```python
from build123d import *

# Parameters (mm, degrees)
SKETCH1_R           = 1.4
BOSS_EXTRUDE1_DEPTH = 2
BOSS_EXTRUDE2_DEPTH = 6


with BuildPart() as part:
    # Sketch1 → Boss-Extrude1 (new body)
    with BuildSketch(Plane.XY):
        with BuildLine():
            Line((78.466333699, 24.25), (60.234282891, 55.828838325))
            ThreePointArc((60.234282891, 55.828838325), (45.078838325, 64.578838325), (29.923393759, 55.828838325))
            Line((29.923393759, 55.828838325), (11.691342951, 24.25))
            ThreePointArc((11.691342951, 24.25), (11.594517635, 6.919891409), (26.455726065, -1.995630053))
            ThreePointArc((26.455726065, -1.995630053), (26.732773023, -2.115865565), (26.846787517, -2.395530168))
            Line((26.846787517, -2.395530168), (26.846787517, -2.834314575))
            ThreePointArc((26.846787517, -2.834314575), (26.81633933, -2.987387948), (26.72963023, -3.117157288))
            Line((26.72963023, -3.117157288), (26.105366161, -3.741421356))
            ThreePointArc((26.105366161, -3.741421356), (26.062011611, -3.806306026), (26.046787517, -3.882842712))
            Line((26.046787517, -3.882842712), (26.046787517, -4))
            ThreePointArc((26.046787517, -4), (26.105366161, -4.141421356), (26.246787517, -4.2))
            Line((26.246787517, -4.2), (63.910889132, -4.2))
            ThreePointArc((63.910889132, -4.2), (64.052310489, -4.141421356), (64.110889132, -4))
            Line((64.110889132, -4), (64.110889132, -3.882842712))
            ThreePointArc((64.110889132, -3.882842712), (64.095665039, -3.806306026), (64.052310489, -3.741421356))
            Line((64.052310489, -3.741421356), (63.42804642, -3.117157288))
            ThreePointArc((63.42804642, -3.117157288), (63.341337319, -2.987387948), (63.310889132, -2.834314575))
            Line((63.310889132, -2.834314575), (63.310889132, -2.395530168))
            ThreePointArc((63.310889132, -2.395530168), (63.424903627, -2.115865565), (63.701950585, -1.995630053))
            ThreePointArc((63.701950585, -1.995630053), (78.563159015, 6.919891409), (78.466333699, 24.25))
        make_face()
        with Locations((65.994459855, 38.101919162)):
            Circle(SKETCH1_R, mode=Mode.SUBTRACT)
        with Locations((45.078838325, 1.875)):
            Circle(SKETCH1_R, mode=Mode.SUBTRACT)
        with Locations((24.163216795, 38.101919162)):
            Circle(SKETCH1_R, mode=Mode.SUBTRACT)
        with BuildLine():
            Line((26.846787517, 10.5), (63.310889132, 10.5))
            ThreePointArc((63.310889132, 10.5), (67.641016151, 13), (67.641016151, 18))
            Line((67.641016151, 18), (49.408965344, 49.578838325))
            ThreePointArc((49.408965344, 49.578838325), (45.078838325, 52.078838325), (40.748711306, 49.578838325))
            Line((40.748711306, 49.578838325), (22.516660498, 18))
            ThreePointArc((22.516660498, 18), (22.516660498, 13), (26.846787517, 10.5))
        make_face(mode=Mode.SUBTRACT)
    extrude(amount=BOSS_EXTRUDE1_DEPTH)

    # Sketch2 → Boss-Extrude2 (add)
    with BuildSketch(Plane(origin=(0, 0, 0), x_dir=(-1, 0, 0), z_dir=(0, 0, -1))):
        with BuildLine():
            ThreePointArc((-27.949498848, 42.516002182), (-45.078838325, 62.398838325), (-62.208177802, 42.516002182))
            ThreePointArc((-62.208177802, 42.516002182), (-63.337010114, 36.567639839), (-67.924026858, 32.615861208))
            ThreePointArc((-67.924026858, 32.615861208), (-76.578398318, 7.84), (-50.794687381, 2.946974934))
            ThreePointArc((-50.794687381, 2.946974934), (-45.078838325, 4.943558647), (-39.362989268, 2.946974934))
            ThreePointArc((-39.362989268, 2.946974934), (-13.579278331, 7.84), (-22.233649792, 32.615861208))
            ThreePointArc((-22.233649792, 32.615861208), (-26.820666536, 36.567639839), (-27.949498848, 42.516002182))
        make_face()
        with BuildLine():
            ThreePointArc((-67.623619549, 31.852870089), (-62.626869283, 36.157639839), (-61.397204455, 42.637337381))
            ThreePointArc((-61.397204455, 42.637337381), (-45.078838325, 61.578838325), (-28.760472195, 42.637337381))
            ThreePointArc((-28.760472195, 42.637337381), (-27.530807367, 36.157639839), (-22.534057101, 31.852870089))
            ThreePointArc((-22.534057101, 31.852870089), (-14.289419162, 8.25), (-38.852423231, 3.588630855))
            ThreePointArc((-38.852423231, 3.588630855), (-45.078838325, 5.763558647), (-51.305253419, 3.588630855))
            ThreePointArc((-51.305253419, 3.588630855), (-75.868257487, 8.25), (-67.623619549, 31.852870089))
        make_face(mode=Mode.SUBTRACT)
    extrude(amount=BOSS_EXTRUDE2_DEPTH)


solid = part.part
```
Geometry check sheet. Reference: the model listing, model coordinates, mm. A direction names the side the tool comes from. Coordinates: 2 decimals unless noted, no trailing zeros. Order: outer loops, then holes, each group sorted by start corner. A loop starts at its lowest first (then second) coordinate and runs counter-clockwise, first axis right, second up.
Item 1: Section check A-A (y = 16.5). Enter the section's corners in (x, z).
Item 2: Depth check by flat-ended pin: pin 1 (4 mm diameter, centred on y = 17.5, z = -1, fed in from +X); pin 2 (2 mm diameter, centred on x = 48, z = 1, fed in from +Y); pin 3 (4 mm diameter, centred on x = 53.5, y = 42.5, fed in from -Z). Enter the tip coordinate at first touch or a pass-through.
Item 3: Section check B-B (x = 37). Enter the section's corners in (y, z), plus the area to 3 significant figures.
Item 4: Mould release check, pull along Y, two halves, no side actions. Record for faces 1 (the flat face through (20.935, 40.26, 0.986)), 2 (the flat face through (29, 31, 2)), 3 (the cylindrical face through (63.294, 36.643, -2.958)): released by +Y, released by -Y, zero draft, split by the parting line, or undercut.
Item 5: Tool access check on faces 4 (the flat face through (48, 2, 0)), 5 (the cylindrical face through (67.604, 12.937, 0.986)), 6 (the cylindrical face through (45.165, 4.943, -2.958)), 7 (the cylindrical face through (78.437, 6.7, 0.986)), 8 (the cylindrical face through (11.472, 7.142, 0.986)). Record the directions out of +Z, -Z, +X, -X, +Y, -Y that give a thin tool (end or side, any length) a straight path to the whole face; none if there is none.
Item 6: Section check D-D (z = 1). Count the separate pieces of the cut face and the enclosed holes in it, plus the area to 3 significant figures.
Item 7: Section check C-C (z = -3.5). Enter the section's corners in (x, y).
Item 8: Scan lines: line 1 along X through (y, z) = (16.5, -4.05); line 2 along X through (y, z) = (3, -0.5); line 3 along X through (y, z) = (31, -1.5). Record each from-to range of solid material in increasing order.
Check sheet entries:
1. outline: (9.38, 0) - (11.26, 0) - (11.26, -6) - (12.08, -6) - (12.08, 0) - (21.95, 0) - (21.95, 2) - (9.38, 2) - close; (68.21, 0) - (78.08, 0) - (78.08, -6) - (78.9, -6) - (78.9, 0) - (80.78, 0) - (80.78, 2) - (68.21, 2) - close
2. pin 1: stops at x = 80.81
2. pin 2: stops at y = 64.47
2. pin 3: stops at z = 0
3. outline: (-4.2, 0) - (1.37, 0) - (1.37, -6) - (2.31, -6) - (2.31, 0) - (10.5, 0) - (10.5, 2) - (-4.2, 2) - close; (43.09, 0) - (59.47, 0) - (59.47, -6) - (60.4, -6) - (60.4, 0) - (62.6, 0) - (62.6, 2) - (43.09, 2) - close
3. area: 79.7 mm2
4. face 1: released by +Y
4. face 2: zero draft
4. face 3: undercut
5. face 4: -Z
5. face 5: +Z, -Z
5. face 6: -Z, -Y
5. face 7: +Z, -Z, +X
5. face 8: +Z, -Z, -X
6. separate pieces: 1
6. enclosed holes: 4
6. area: 2,310 mm2
7. outline: (22.23, 32.62) arc R17.32 ccw (long way) to (39.36, 2.95) arc R9.18 cw to (50.79, 2.95) arc R17.32 ccw (long way) to (67.92, 32.62) arc R9.18 cw to (62.21, 42.52) arc R17.32 ccw (long way) to (27.95, 42.52) arc R9.18 cw to start; hole (22.53, 31.85) arc R16.5 ccw (long way) to (38.85, 3.59) arc R10 cw to (51.31, 3.59) arc R16.5 ccw (long way) to (67.62, 31.85) arc R10 cw to (61.4, 42.64) arc R16.5 ccw (long way) to (28.76, 42.64) arc R10 cw to start
8. line 1: x = 11.26 to 12.08, 78.08 to 78.9
8. line 2: x = 17.73 to 19.09, 38.07 to 39.43, 50.73 to 52.09, 71.07 to 72.43
8. line 3: x = 19.11 to 20.7, 69.45 to 71.05
